Geometry check sheet. Reference: the model listing, model coordinates, mm. A direction names the side the tool comes from. Round coordinates to 2 decimals unless told otherwise and drop trailing zeros. Loops run counter-clockwise (first coordinate to the right, second up) from the corner with the lowest first, then second, coordinate; pieces in that order, holes last.
```python
from build123d import *

# Parameters (mm, degrees)
SKETCH1_R           = 1.5
BOSS_EXTRUDE1_DEPTH = 6.35
FILLET1_R           = 2
SKETCH2_R           = 1.5
CUT_EXTRUDE1_DEPTH  = 7.35


with BuildPart() as part:
    # Sketch1 → Boss-Extrude1 (new body)
    with BuildSketch(Plane(origin=(0, 0, 0), x_dir=(1, 0, 0), z_dir=(0, 1, 0))):
        Polygon((-32.64725, 32.8), (30.21585, 32.8), (30.21585, -33.654999237), (13.81125, -33.654999237), (13.81125, -44), (34.38525, -44), (34.38525, 44), (9.70725, 44), (9.70725, 40.8), (-5.72675, 40.8), (-5.72675, 44), (-62.13475, 44), (-62.13475, -44), (-41.56075, -44), (-41.56075, -33.654999237), (-56.51475, -33.654999237), (-56.51475, 32.8), (-44.33475, 32.8), (-44.33475, 42.8), (-32.64725, 42.8), align=None)
        with Locations((-52.38475, -35.75)):
            Circle(SKETCH1_R, mode=Mode.SUBTRACT)
        with Locations((19.11525, -35.75)):
            Circle(SKETCH1_R, mode=Mode.SUBTRACT)
        with Locations((-52.38475, 35.75)):
            Circle(SKETCH1_R, mode=Mode.SUBTRACT)
        with Locations((-20.38475, 35.75)):
            Circle(SKETCH1_R, mode=Mode.SUBTRACT)
        with Locations((19.11525, 35.75)):
            Circle(SKETCH1_R, mode=Mode.SUBTRACT)
        with BuildLine():
            Line((34.38525, -44), (13.81125, -44))
            Line((13.81125, -44), (13.81125, -48.259999237))
            Line((13.81125, -48.259999237), (-41.56075, -48.259999237))
            Line((-41.56075, -48.259999237), (-41.56075, -44))
            Line((-41.56075, -44), (-62.13475, -44))
            Line((-62.13475, -44), (-62.13475, -48.768))
            ThreePointArc((-62.13475, -48.768), (-61.539590979, -50.204840979), (-60.10275, -50.8))
            Line((-60.10275, -50.8), (32.35325, -50.8))
            ThreePointArc((32.35325, -50.8), (33.790090979, -50.204840979), (34.38525, -48.768))
            Line((34.38525, -48.768), (34.38525, -44))
        make_face()
        with BuildLine():
            Line((-62.13475, 48.768), (-62.13475, 44))
            Line((-62.13475, 44), (-5.72675, 44))
            Line((-5.72675, 44), (-5.72675, 50.8))
            Line((-5.72675, 50.8), (-60.10275, 50.8))
            ThreePointArc((-60.10275, 50.8), (-61.539590979, 50.204840979), (-62.13475, 48.768))
        make_face()
        with BuildLine():
            Line((9.70725, 44), (34.38525, 44))
            Line((34.38525, 44), (34.38525, 48.768))
            ThreePointArc((34.38525, 48.768), (33.790090979, 50.204840979), (32.35325, 50.8))
            Line((32.35325, 50.8), (9.70725, 50.8))
            Line((9.70725, 50.8), (9.70725, 44))
        make_face()
        with BuildLine():
            Line((34.38525, 48.768), (34.38525, 44))
            Line((34.38525, 44), (60.86525, 44))
            Line((60.86525, 44), (60.86525, 50.8))
            Line((60.86525, 50.8), (32.35325, 50.8))
            ThreePointArc((32.35325, 50.8), (33.790090979, 50.204840979), (34.38525, 48.768))
        make_face()
        Polygon((34.38525, 44), (34.38525, -44), (60.86525, -44), (60.86525, -13.081), (35.97275, -13.081), (35.97275, 13.081), (60.86525, 13.081), (60.86525, 44), align=None)
        with Locations((51.11525, -35.75)):
            Circle(SKETCH1_R, mode=Mode.SUBTRACT)
        with Locations((51.11525, 35.75)):
            Circle(SKETCH1_R, mode=Mode.SUBTRACT)
        with BuildLine():
            Line((60.86525, -44), (34.38525, -44))
            Line((34.38525, -44), (34.38525, -48.768))
            ThreePointArc((34.38525, -48.768), (33.790090979, -50.204840979), (32.35325, -50.8))
            Line((32.35325, -50.8), (60.86525, -50.8))
            Line((60.86525, -50.8), (60.86525, -44))
        make_face()
    extrude(amount=BOSS_EXTRUDE1_DEPTH)

    # Fillet1
    fillet1_edges = [part.edges().sort_by_distance(p)[0] for p in [
        (60.86525, 3.175, -50.8),
        (60.86525, 3.175, 50.8),
        (30.21585, 3.175, 33.654999237),
        (30.21585, 3.175, -32.8),
        (-56.51475, 3.175, -32.8),
        (-56.51475, 3.175, 33.654999237),
        (-41.56075, 3.175, 48.259999237),
        (13.81125, 3.175, 48.259999237),
    ]]
    fillet(fillet1_edges, radius=FILLET1_R)

    # Sketch2 → Cut-Extrude1 (cut, through all)
    with BuildSketch(Plane(origin=(0, 6.35, 0), x_dir=(1, 0, 0), z_dir=(0, 1, 0))):
        with Locations((-59.79712037, -48.3933723)):
            Circle(SKETCH2_R)
        with Locations((32.04762038, -48.3933723)):
            Circle(SKETCH2_R)
        with Locations((32.04762038, 48.28530217)):
            Circle(SKETCH2_R)
        with Locations((-59.79712037, 48.28530217)):
            Circle(SKETCH2_R)
    extrude(amount=-CUT_EXTRUDE1_DEPTH, mode=Mode.SUBTRACT)


solid = part.part
```
1) Gauge pin test, flat end, axial feed: pin 1 (2.5 mm diameter, centred on x = 19.12, z = 35.75, fed in from -Y). Record the tip position at first contact, or that the pin passes through.
Report:
pin 1: passes through
2) Access from +Z, -Z, +X, -X, +Y, -Y to the whole of each face (thin tool, end or side, straight path). Record for faces 1 (the face through (35, 3, -50.8)), 2 (the face through (21, 3, 33.655)), 3 (the face through (49, 3, 13.081)).
Report:
face 1: -Z, +X, -X, +Y, -Y
face 2: +Y, -Y
face 3: +X, +Y, -Y
3) Sectioned sample at B-B, the plane z = -35.75. Record the cut outline in (x, y), then the cut area to 3 significant figures.
Report:
outline: (-62.13, 0) - (-53.88, 0) - (-53.88, 6.35) - (-62.13, 6.35) - close; (-50.88, 0) - (-44.33, 0) - (-44.33, 6.35) - (-50.88, 6.35) - close; (-32.65, 0) - (-21.88, 0) - (-21.88, 6.35) - (-32.65, 6.35) - close; (-18.88, 0) - (17.62, 0) - (17.62, 6.35) - (-18.88, 6.35) - close; (20.62, 0) - (49.62, 0) - (49.62, 6.35) - (20.62, 6.35) - close; (52.62, 0) - (60.87, 0) - (60.87, 6.35) - (52.62, 6.35) - close
area: 631 mm2
4) Scan lines: line 1 along X through (y, z) = (3.25, 35.75); line 2 along X through (y, z) = (2.75, -35.75); line 3 along Z through (x, y) = (-31.5, 4.5). Record each from-to range of solid material in increasing order.
Report:
line 1: x = -62.13 to -53.88, -50.88 to -41.56, 13.81 to 17.62, 20.62 to 49.62, 52.62 to 60.87
line 2: x = -62.13 to -53.88, -50.88 to -44.33, -32.65 to -21.88, -18.88 to 17.62, 20.62 to 49.62, 52.62 to 60.87
line 3: z = -50.8 to -32.8, 48.26 to 50.8
5) Mould release check, pull along X, two halves, no side actions. Record for faces 4 (the face through (60.865, 3, 31)), 5 (the face through (-33, 3, -50.8)), 6 (the face through (-19.69, 3.13, -34.42)): +X half, -X half, draft (parallel to the pull), parting line (faces both ways), or undercut.
Report:
face 4: +X half
face 5: draft
face 6: undercut
6) Sectioned sample at D-D, the plane x = 42.5. Record the cut outline in (y, z), then the cut area to 3 significant figures.
Report:
outline: (0, -50.8) - (6.35, -50.8) - (6.35, -13.08) - (0, -13.08) - close; (0, 13.08) - (6.35, 13.08) - (6.35, 50.8) - (0, 50.8) - close
area: 479 mm2
7) Sectioned sample at A-A, the plane x = -36. Record the cut outline in (y, z), then the cut area to 3 significant figures.
Report:
outline: (0, -50.8) - (6.35, -50.8) - (6.35, -42.8) - (0, -42.8) - close; (0, 48.26) - (6.35, 48.26) - (6.35, 50.8) - (0, 50.8) - close
area: 66.9 mm2
8) Sectioned sample at C-C, the plane z = 35.75. Record the cut outline in (x, y), then the cut area to 3 significant figures.
Report:
outline: (-62.13, 0) - (-53.88, 0) - (-53.88, 6.35) - (-62.13, 6.35) - close; (-50.88, 0) - (-41.56, 0) - (-41.56, 6.35) - (-50.88, 6.35) - close; (13.81, 0) - (17.62, 0) - (17.62, 6.35) - (13.81, 6.35) - close; (20.62, 0) - (49.62, 0) - (49.62, 6.35) - (20.62, 6.35) - close; (52.62, 0) - (60.87, 0) - (60.87, 6.35) - (52.62, 6.35) - close
area: 372 mm2
